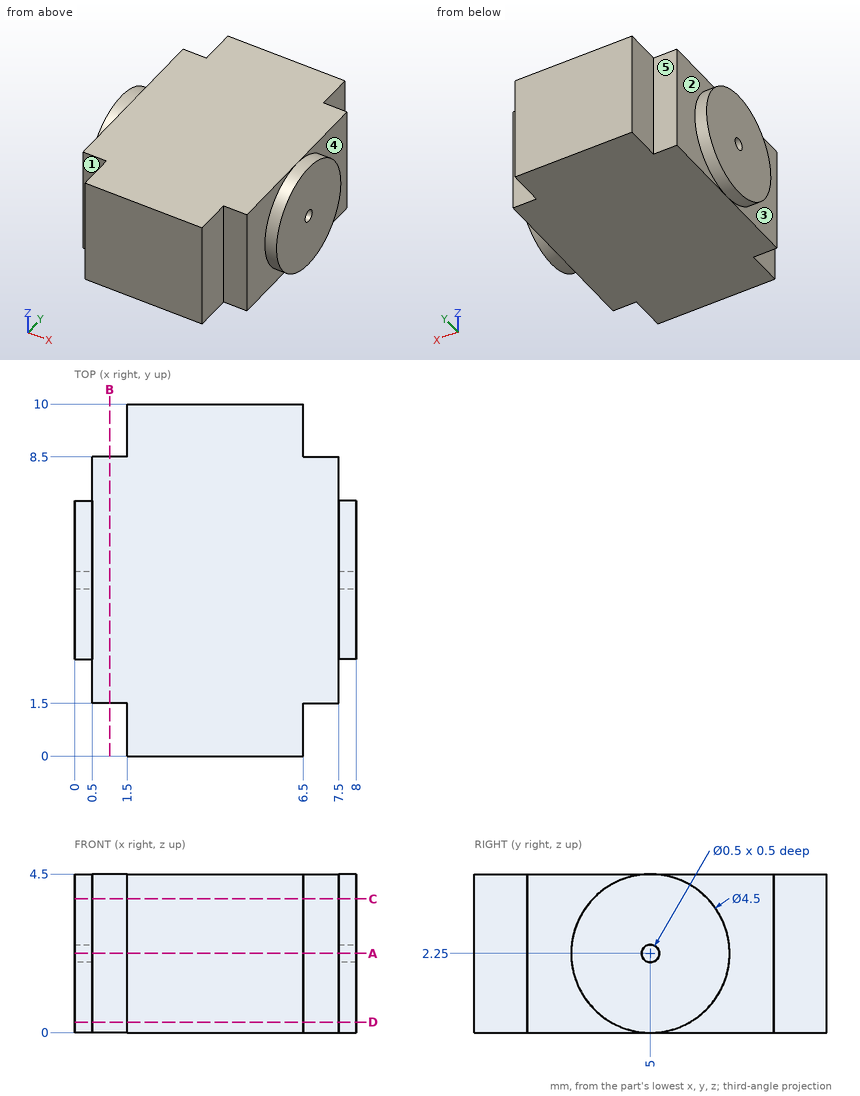
Answer from the drawing. Dimensions are ordinates in mm from the lowest x, y and z of the part. A direction names the side the tool comes from. Coordinates: 2 decimals unless noted, no trailing zeros. Write each loop counter-clockwise with the first axis right and the second up, starting at its lowest first coordinate (ties: lowest second). Pieces come first, ordered by that corner, then holes. Notation, with made-up numbers: (7.5, -10) - (29.5, -10) arc R24 cw to (29.5, 5) - close; hole circle Ø4 at (-7, 20). An arc over 180 degrees is marked (long way). Return JSON: item names as keys, results as strings.
1. The part is cut by section A-A on z = 2.25. Determine the outline of the cut face in (x, y).
Final values:
{"outline": "(0, 2.75) - (0.5, 2.75) - (0.5, 1.5) - (1.5, 1.5) - (1.5, 0) - (6.5, 0) - (6.5, 1.5) - (7.5, 1.5) - (7.5, 2.75) - (8, 2.75) - (8, 4.75) - (7.5, 4.75) - (7.5, 5.25) - (8, 5.25) - (8, 7.25) - (7.5, 7.25) - (7.5, 8.5) - (6.5, 8.5) - (6.5, 10) - (1.5, 10) - (1.5, 8.5) - (0.5, 8.5) - (0.5, 7.25) - (0, 7.25) - (0, 5.25) - (0.5, 5.25) - (0.5, 4.75) - (0, 4.75) - close"}
2. Each of these flat-tipped pins is pushed along its axis until it touches: pin 1 Ø0.8 at (x, z) = (1, 3) entering from -Y; pin 2 Ø1.2 at (y, z) = (1, 1.5) entering from -X; pin 3 Ø1.6 at (y, z) = (9, 1.5) entering from +X. Where does it stop, or does it pass through?
Final values:
{"pin 1": "y = 1.5", "pin 2": "x = 0.5", "pin 3": "x = 7.5"}
3. Consider line 1 along Y through (x, z) = (0.45, 2.25); line 2 along X through (y, z) = (1, 2.2); line 3 along X through (y, z) = (7.5, 2.15). Determine where each line is inside the solid, lowest interval first.
Final values:
{"line 1": "2.75 to 4.75, 5.25 to 7.25", "line 2": "1.5 to 6.5", "line 3": "0.5 to 7.5"}
4. The part is cut by section B-B on x = 1. Determine the outline of the cut face in (y, z).
Final values:
{"outline": "(1.5, 0) - (8.5, 0) - (8.5, 4.5) - (1.5, 4.5) - close"}
5. The part is cut by section C-C on z = 3.8. Determine the outline of the cut face in (x, y), then the cut area to 3 significant figures.
Final values:
{"outline": "(0, 3.37) - (0.5, 3.37) - (0.5, 1.5) - (1.5, 1.5) - (1.5, 0) - (6.5, 0) - (6.5, 1.5) - (7.5, 1.5) - (7.5, 3.37) - (8, 3.37) - (8, 6.63) - (7.5, 6.63) - (7.5, 8.5) - (6.5, 8.5) - (6.5, 10) - (1.5, 10) - (1.5, 8.5) - (0.5, 8.5) - (0.5, 6.63) - (0, 6.63) - close", "area": "67.3 mm^2"}
6. Which of the six approach directions +Z, -Z, +X, -X, +Y, -Y give full straight-line access (tool end or side, diameter ignored) to the marked faces 1, 2, 3, 4 and 5?
Final values:
{"face 1": "+Z, -Z, -X, -Y", "face 2": "-X, +Y", "face 3": "-X, -Y", "face 4": "+X, +Y", "face 5": "+Z, -Z, -X, +Y"}
7. The part is cut by section D-D on z = 0.3. Determine the outline of the cut face in (x, y).
Final values:
{"outline": "(0, 3.88) - (0.5, 3.88) - (0.5, 1.5) - (1.5, 1.5) - (1.5, 0) - (6.5, 0) - (6.5, 1.5) - (7.5, 1.5) - (7.5, 3.88) - (8, 3.88) - (8, 6.12) - (7.5, 6.12) - (7.5, 8.5) - (6.5, 8.5) - (6.5, 10) - (1.5, 10) - (1.5, 8.5) - (0.5, 8.5) - (0.5, 6.12) - (0, 6.12) - close"}
